Work out the finished part from the listing and answer in its coordinate system (mm). Give positions to 0.01 mm unless a question says otherwise; leave off trailing zeros. Write each loop counter-clockwise with the first axis right and the second up, starting at its lowest first coordinate (ties: lowest second). Pieces come first, ordered by that corner, then holes. Notation, with made-up numbers: (38, 19) - (79, 19) arc R16 cw to (79, 32) - close; hole circle Ø7 at (39.5, 20.5). An arc over 180 degrees is marked (long way). Write each question's results on one line, items separated by ' | '. Start each with the question number.
from build123d import *

# Parameters (mm, degrees)
F0_W     = 93.98
F0_H     = 68.58
F1_DEPTH = 2.54
F2_W     = 88.392
F2_H     = 62.992
F3_DEPTH = 1.524
F4_W     = 12.7
F4_H     = 43.18
F5_DEPTH = 4.065
F6_W     = 20.32
F6_H     = 43.18
F7_DEPTH = 4.065


# Not quite as in the source:
# - a feature names something its author has since deleted; it is built from what else it names


with BuildPart() as f1:
    # F0 (on Top) → F1 (new body)
    with BuildSketch(Plane.XY):
        with Locations((-1.1547841132, -14.7677313863)):
            Rectangle(F0_W, F0_H)
    extrude(amount=F1_DEPTH)

    # F2 (on face) → F3 (join)
    with BuildSketch(Plane.XY.offset(2.54)):
        with Locations((-1.1547841132, -14.7677313863)):
            Rectangle(F2_W, F2_H)
    extrude(amount=F3_DEPTH)

    # F4 (on face) → F5 (cut, through all)
    with BuildSketch(Plane.XY.offset(4.064)):
        with Locations((30.5952158868, -14.5137313863)):
            Rectangle(F4_W, F4_H)
    extrude(amount=-F5_DEPTH, mode=Mode.SUBTRACT)

    # F6 (on face) → F7 (cut, through all)
    with BuildSketch(Plane.XY.offset(4.064)):
        with Locations((-30.3647841132, -14.5137313863)):
            Rectangle(F6_W, F6_H)
    extrude(amount=-F7_DEPTH, mode=Mode.SUBTRACT)


solid = f1.part
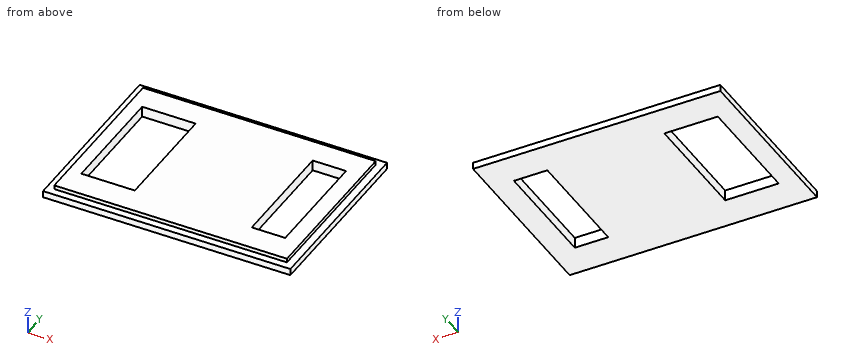
Q1. A cutting plane is placed at C-C, the plane z = 1.8. Write down the section's boundary in (x, y), and give its area (3 significant figures).
Q2. A cutting plane is placed at D-D, the plane x = -41.5. Write down the section's boundary in (y, z), and give its area (3 significant figures).
Q3. A cutting plane is placed at B-B, the plane x = -23.5. Write down the section's boundary in (y, z).
Q4. Given pin 1 (1.5 mm diameter, centred on x = -36.5, z = 3.5, fed in from +Y); pin 2 (1 mm diameter, centred on x = -22, y = -17, fed in from +Z); pin 3 (0.5 mm diameter, centred on x = -6, z = 3, fed in from -Y); pin 4 (0.5 mm diameter, centred on y = -26, z = 3, fed in from -X), each flat-ended and moving along its own axis, determine where each tip first touches the part or whether it passes through.
Q5. Consider L1, parallel to X at y = -15, z = 0.7; L2, parallel to Y at x = -31, z = 3.05; L3, parallel to Y at x = -2, z = 3.35. Determine where each line is inside the solid, lowest interval first.
Q6. A cutting plane is placed at A-A, the plane y = -9. Write down the section's boundary in (x, z).
Result:
1) outline: (-48.14, -49.06) - (45.84, -49.06) - (45.84, 19.52) - (-48.14, 19.52) - close; hole (-40.52, -36.1) - (-20.2, -36.1) - (-20.2, 7.08) - (-40.52, 7.08) - close; hole (24.25, -36.1) - (36.95, -36.1) - (36.95, 7.08) - (24.25, 7.08) - close | area: 5,020 mm2
2) outline: (-49.06, 0) - (19.52, 0) - (19.52, 2.54) - (16.73, 2.54) - (16.73, 4.06) - (-46.26, 4.06) - (-46.26, 2.54) - (-49.06, 2.54) - close | area: 270 mm2
3) outline: (-49.06, 0) - (-36.1, 0) - (-36.1, 4.06) - (-46.26, 4.06) - (-46.26, 2.54) - (-49.06, 2.54) - close; (7.08, 0) - (19.52, 0) - (19.52, 2.54) - (16.73, 2.54) - (16.73, 4.06) - (7.08, 4.06) - close
4) pin 1: stops at y = 16.73 | pin 2: passes through | pin 3: stops at y = -46.26 | pin 4: stops at x = -45.35
5) L1: x = -48.14 to -40.52, -20.2 to 24.25, 36.95 to 45.84 | L2: y = -46.26 to -36.1, 7.08 to 16.73 | L3: y = -46.26 to 16.73
6) outline: (-48.14, 0) - (-40.52, 0) - (-40.52, 4.06) - (-45.35, 4.06) - (-45.35, 2.54) - (-48.14, 2.54) - close; (-20.2, 0) - (24.25, 0) - (24.25, 4.06) - (-20.2, 4.06) - close; (36.95, 0) - (45.84, 0) - (45.84, 2.54) - (43.04, 2.54) - (43.04, 4.06) - (36.95, 4.06) - close
